Input: part model. Units: mm. Frame: model coordinates. Face numbers are marked on the shaded views. A direction names the side the tool comes from. Coordinates: 2 decimals unless noted, no trailing zeros. Order: outer loops, then holes, each group sorted by start corner. A loop starts at its lowest first (then second) coordinate and runs counter-clockwise, first axis right, second up.
from build123d import *

# Parameters (mm, degrees)
SKETCH_1_W           = 102
SKETCH_1_H           = 54
SKETCH_1_W_2         = 44
SKETCH_1_H_2         = 44
EXTRUDE_1_DEPTH      = 5
SKETCH_2_W           = 102
SKETCH_2_H           = 54
SKETCH_2_W_2         = 98
SKETCH_2_H_2         = 49.988098762
SKETCH_2_W_3         = 44
SKETCH_2_H_3         = 44
SKETCH_2_W_4         = 39.827305616
SKETCH_2_H_4         = 40.011901238
EXTRUDE_2_DEPTH      = 3
SKETCH_3_W           = 106
SKETCH_3_H           = 106
SKETCH_3_W_2         = 102
SKETCH_3_H_2         = 102
EXTRUDE_3_DEPTH      = 30
SKETCH_4_W           = 12
SKETCH_4_H           = 10
SKETCH_4_H_2         = 13
CUT_EXTRUDE_1_DEPTH  = 30
SKETCH_5_W           = 44
SKETCH_5_H           = 44
CUT_EXTRUDE_2_DEPTH  = 3
SKETCH_6_W           = 39.675099194
SKETCH_6_H           = 39.248485224
CUT_EXTRUDE_3_DEPTH  = 87.290021993
SKETCH_8_W           = 39.827305616
SKETCH_8_H           = 40.011901238
SKETCH_8_W_2         = 7.107215528
SKETCH_8_H_2         = 49.988098762
EXTRUDE_5_DEPTH      = 2
EXTRUDE_6_DEPTH      = 2
EXTRUDE_6_DEPTH_BACK = 3
SKETCH_9_W           = 44
SKETCH_9_H           = 44
SKETCH_10_W          = 44
SKETCH_10_H          = 44
CUT_EXTRUDE_5_DEPTH  = 3
SKETCH_11_W          = 39.141831732
SKETCH_11_H          = 39.141831732
CUT_EXTRUDE_6_DEPTH  = 3
SKETCH_12_W          = 10
SKETCH_12_H          = 30
EXTRUDE_7_DEPTH      = 10
SKETCH_13_W          = 3.5
SKETCH_13_H          = 24
CUT_EXTRUDE_7_DEPTH  = 20
CUT_EXTRUDE_8_DEPTH  = 29.999730027
SKETCH_15_W          = 15.5
SKETCH_15_H          = 20.5
CUT_EXTRUDE_9_DEPTH  = 30
SKETCH_18_W          = 102
SKETCH_18_H          = 48
CUT_EXTRUDE_11_DEPTH = 2
CUT_EXTRUDE_12_DEPTH = 124.099226215
EXTRUDE_10_DEPTH     = 6
SKETCH_21_R          = 2
EXTRUDE_11_DEPTH     = 3


with BuildPart() as part:
    # 草图1 → 凸台-拉伸1 (new body)
    with BuildSketch(Plane.XY):
        Polygon((-56.9609375, 55.7890625), (49.0390625, 55.7890625), (49.0390625, -2.2109375), (49.0390625, -50.2109375), (-8.9609375, -50.2109375), (-56.9609375, -50.2109375), (-56.9609375, -2.2109375), align=None)
        with Locations((-3.9609375, 26.7890625)):
            Rectangle(SKETCH_1_W, SKETCH_1_H, mode=Mode.SUBTRACT)
        with Locations((-32.9609375, -26.2109375)):
            Rectangle(SKETCH_1_W_2, SKETCH_1_H_2, mode=Mode.SUBTRACT)
    extrude(amount=EXTRUDE_1_DEPTH)

    # 草图2 → 凸台-拉伸2 (add)
    # profile 1 of 2: a face of its own
    with BuildSketch(Plane(origin=(0, 0, 0), x_dir=(-1, 0, 0), z_dir=(0, 0, -1))):
        with Locations((3.9609375, 26.7890625)):
            Rectangle(SKETCH_2_W, SKETCH_2_H)
        with Locations((3.9609375, 26.795013119)):
            Rectangle(SKETCH_2_W_2, SKETCH_2_H_2, mode=Mode.SUBTRACT)
    # profile 2 of 2: a face of its own
    with BuildSketch(Plane(origin=(0, 0, 0), x_dir=(-1, 0, 0), z_dir=(0, 0, -1))):
        with Locations((32.9609375, -26.2109375)):
            Rectangle(SKETCH_2_W_3, SKETCH_2_H_3)
        with Locations((33.047284692, -26.204986881)):
            Rectangle(SKETCH_2_W_4, SKETCH_2_H_4, mode=Mode.SUBTRACT)
    extrude(amount=-EXTRUDE_2_DEPTH)

    # 草图3 → 凸台-拉伸3 (add)
    with BuildSketch(Plane.XY.offset(5)):
        with Locations((-3.9609375, 2.7890625)):
            Rectangle(SKETCH_3_W, SKETCH_3_H)
        with Locations((-3.9609375, 2.7890625)):
            Rectangle(SKETCH_3_W_2, SKETCH_3_H_2, mode=Mode.SUBTRACT)
    extrude(amount=EXTRUDE_3_DEPTH)

    # 草图4 → 切除-拉伸1 (cut)
    with BuildSketch(Plane(origin=(49.0390625, 0, 0), x_dir=(0, 0, -1), z_dir=(1, 0, 0))):
        with Locations((-9, 44.531190652)):
            Rectangle(SKETCH_4_W, SKETCH_4_H)
        with Locations((-9, 13.608528945)):
            Rectangle(SKETCH_4_W, SKETCH_4_H_2)
    extrude(amount=-CUT_EXTRUDE_1_DEPTH, mode=Mode.SUBTRACT)

    # 草图5 → 切除-拉伸2 (cut)
    with BuildSketch(Plane.XY.offset(5)):
        with Locations((18.871191973, -24.065672965)):
            Rectangle(SKETCH_5_W, SKETCH_5_H)
    extrude(amount=-CUT_EXTRUDE_2_DEPTH, mode=Mode.SUBTRACT)

    # 草图6 → 切除-拉伸3 (cut, through all)
    with BuildSketch(Plane.XY.offset(2)):
        with Locations((19.129543617, -24.247597838)):
            Rectangle(SKETCH_6_W, SKETCH_6_H)
    extrude(amount=-CUT_EXTRUDE_3_DEPTH, mode=Mode.SUBTRACT)

    # 草图8 → 凸台-拉伸5 (add)
    with BuildSketch(Plane(origin=(0, 0, 0), x_dir=(-1, 0, 0), z_dir=(0, 0, -1))):
        with Locations((33.047284692, -26.204986881)):
            Rectangle(SKETCH_8_W, SKETCH_8_H)
        with Locations((3.553607764, 26.795013119)):
            Rectangle(SKETCH_8_W_2, SKETCH_8_H_2)
    extrude(amount=-EXTRUDE_5_DEPTH)

    # 草图9 → 凸台-拉伸6 (add, two sides: drawn at the far end of the back side and taken through both)
    with BuildSketch(Plane.XY.offset(3).offset(-EXTRUDE_6_DEPTH_BACK)):
        with Locations((-32.9609375, -26.2109375)):
            Rectangle(SKETCH_9_W, SKETCH_9_H)
    extrude(amount=EXTRUDE_6_DEPTH + EXTRUDE_6_DEPTH_BACK)

    # 草图10 → 切除-拉伸5 (cut)
    with BuildSketch(Plane.XY.offset(5)):
        with Locations((-27.400759648, -24.065672965)):
            Rectangle(SKETCH_10_W, SKETCH_10_H)
    extrude(amount=-CUT_EXTRUDE_5_DEPTH, mode=Mode.SUBTRACT)

    # 草图11 → 切除-拉伸6 (cut)
    with BuildSketch(Plane.XY.offset(2)):
        with Locations((-27.424705841, -24.087617599)):
            Rectangle(SKETCH_11_W, SKETCH_11_H)
    extrude(amount=-CUT_EXTRUDE_6_DEPTH, mode=Mode.SUBTRACT)

    # 草图12 → 凸台-拉伸7 (add)
    with BuildSketch(Plane(origin=(49.0390625, 0, 0), x_dir=(0, 0, -1), z_dir=(1, 0, 0))):
        with Locations((-25.778359811, 38.789332473)):
            Rectangle(SKETCH_12_W, SKETCH_12_H)
    extrude(amount=-EXTRUDE_7_DEPTH)

    # 草图13 → 切除-拉伸7 (cut)
    with BuildSketch(Plane(origin=(49.0390625, 0, 0), x_dir=(0, 0, -1), z_dir=(1, 0, 0))):
        with Locations((-27.833078142, 37.536383555)):
            Rectangle(SKETCH_13_W, SKETCH_13_H)
    extrude(amount=-CUT_EXTRUDE_7_DEPTH, mode=Mode.SUBTRACT)

    # 草图14 → 切除-拉伸8 (cut)
    with BuildSketch(Plane.XZ.offset(-23.789332473)):
        Polygon((37.906859467, 25.472396685), (38.543242323, 25.472396685), (47.0390625, 20.778359811), (47.0390625, 19.400243598), (37.906859467, 19.400243598), align=None)
    extrude(amount=-CUT_EXTRUDE_8_DEPTH, mode=Mode.SUBTRACT)

    # 草图15 → 切除-拉伸9 (cut)
    with BuildSketch(Plane(origin=(49.0390625, 0, 0), x_dir=(0, 0, -1), z_dir=(1, 0, 0))):
        with Locations((-24.841469183, 4.666763342)):
            Rectangle(SKETCH_15_W, SKETCH_15_H)
    extrude(amount=-CUT_EXTRUDE_9_DEPTH, mode=Mode.SUBTRACT)

    # 草图18 → 切除-拉伸11 (cut)
    with BuildSketch(Plane.XY.offset(5)):
        with Locations((-3.9609375, -24.2109375)):
            Rectangle(SKETCH_18_W, SKETCH_18_H)
    extrude(amount=-CUT_EXTRUDE_11_DEPTH, mode=Mode.SUBTRACT)

    # 草图19 → 切除-拉伸12 (cut, through all)
    with BuildSketch(Plane(origin=(-54.9609375, 0, 0), x_dir=(0, 0, -1), z_dir=(1, 0, 0))):
        with BuildLine():
            Line((-8, -9.636069371), (-6, -9.636069371))
            ThreePointArc((-6, -9.636069371), (-3.878679656, -10.514749028), (-3, -12.636069371))
            Line((-3, -12.636069371), (-3, -36.636069371))
            ThreePointArc((-3, -36.636069371), (-3.878679656, -38.757389715), (-6, -39.636069371))
            Line((-6, -39.636069371), (-8, -39.636069371))
            ThreePointArc((-8, -39.636069371), (-10.121320344, -38.757389715), (-11, -36.636069371))
            Line((-11, -36.636069371), (-11, -12.636069371))
            ThreePointArc((-11, -12.636069371), (-10.121320344, -10.514749028), (-8, -9.636069371))
        make_face()
    extrude(amount=-CUT_EXTRUDE_12_DEPTH, mode=Mode.SUBTRACT)

    # 草图20 → 凸台-拉伸10 (add)
    with BuildSketch(Plane.ZY.offset(56.9609375)):
        with BuildLine():
            Line((3, -36.636069371), (3, -41.845424094))
            Line((3, -41.845424094), (9.180533555, -41.845424094))
            ThreePointArc((9.180533555, -41.845424094), (12.00896068, -40.673851218), (13.180533555, -37.845424094))
            Line((13.180533555, -37.845424094), (13.180533555, -11.076385552))
            ThreePointArc((13.180533555, -11.076385552), (12.00896068, -8.247958428), (9.180533555, -7.076385552))
            Line((9.180533555, -7.076385552), (3, -7.076385552))
            Line((3, -7.076385552), (3, -12.636069371))
            ThreePointArc((3, -12.636069371), (3.878679656, -10.514749028), (6, -9.636069371))
            Line((6, -9.636069371), (8, -9.636069371))
            ThreePointArc((8, -9.636069371), (10.121320344, -10.514749028), (11, -12.636069371))
            Line((11, -12.636069371), (11, -36.636069371))
            ThreePointArc((11, -36.636069371), (10.121320344, -38.757389715), (8, -39.636069371))
            Line((8, -39.636069371), (6, -39.636069371))
            ThreePointArc((6, -39.636069371), (3.878679656, -38.757389715), (3, -36.636069371))
        make_face()
        Polygon((0, -7.076385552), (0, -41.845424094), (3, -41.845424094), (3, -36.636069371), (3, -12.636069371), (3, -7.076385552), align=None)
    extrude(amount=EXTRUDE_10_DEPTH)

    # 草图21 → 凸台-拉伸11 (add)
    # profile 1 of 2: a face of its own
    with BuildSketch(Plane(origin=(0, 0, 0), x_dir=(-1, 0, 0), z_dir=(0, 0, -1))):
        with BuildLine():
            Line((56.9609375, -2.916899347), (64.873289872, -2.916899347))
            ThreePointArc((64.873289872, -2.916899347), (67.701716997, -1.745326471), (68.873289872, 1.083100653))
            Line((68.873289872, 1.083100653), (68.873289872, 4.495024347))
            ThreePointArc((68.873289872, 4.495024347), (67.701716997, 7.323451471), (64.873289872, 8.495024347))
            Line((64.873289872, 8.495024347), (56.9609375, 8.495024347))
            Line((56.9609375, 8.495024347), (56.9609375, -2.916899347))
        make_face()
        with Locations((62.900694294, 2.7890625)):
            Circle(SKETCH_21_R, mode=Mode.SUBTRACT)
    # profile 2 of 2: a face of its own
    with BuildSketch(Plane(origin=(0, 0, 0), x_dir=(-1, 0, 0), z_dir=(0, 0, -1))):
        with BuildLine():
            Line((-60.951414872, 1.083100653), (-60.951414872, 4.495024347))
            ThreePointArc((-60.951414872, 4.495024347), (-59.779841997, 7.323451471), (-56.951414872, 8.495024347))
            Line((-56.951414872, 8.495024347), (-49.0390625, 8.495024347))
            Line((-49.0390625, 8.495024347), (-49.0390625, -2.916899347))
            Line((-49.0390625, -2.916899347), (-56.951414872, -2.916899347))
            ThreePointArc((-56.951414872, -2.916899347), (-59.779841997, -1.745326471), (-60.951414872, 1.083100653))
        make_face()
        with Locations(Location((-54.978819294, 2.7890625, 0), (0, 0, 180))):
            Circle(SKETCH_21_R, mode=Mode.SUBTRACT)
    extrude(amount=-EXTRUDE_11_DEPTH)


solid = part.part
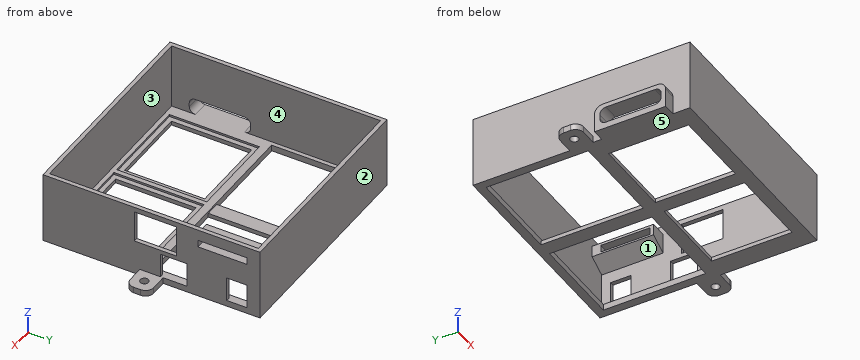
Item 1: Ray query, probe 1 along X at (y, z) = (-19, 29.5); probe 2 along Y at (x, z) = (27.5, 29); probe 3 along X at (y, z) = (32, 26). Return the intervals inside material, ascending.
Response values:
probe 1: x = -56.96 to -54.96, 47.04 to 49.04
probe 2: y = -50.21 to -48.21, 53.79 to 55.79
probe 3: x = -56.96 to -54.96, 39.04 to 49.04
Item 2: Pin query (flat end, axial travel): pin 1 Ø6 at (y, z) = (-24, 26) entering from -X; pin 2 Ø3.5 at (x, z) = (-59.5, 1.5) entering from -Y; pin 3 Ø2 at (y, z) = (-30.5, 8.5) entering from -X. Return the tip coordinate at first contact, or that it passes through.
Response values:
pin 1: stops at x = -56.96
pin 2: stops at y = -41.85
pin 3: stops at x = 47.04
Item 3: Cut plane A-A on x = -13. Return loops of the section in (y, z).
Response values:
outline: (-50.21, 0) - (-43.66, 0) - (-43.66, 2) - (-46.07, 2) - (-46.07, 3) - (-48.21, 3) - (-48.21, 35) - (-50.21, 35) - close; (-4.52, 0) - (1.8, 0) - (1.8, 3) - (-2.07, 3) - (-2.07, 2) - (-4.52, 2) - close; (51.79, 0) - (55.79, 0) - (55.79, 35) - (53.79, 35) - (53.79, 3) - (51.79, 3) - close
Item 4: Draft query along X for the marked faces 4 and 5. Return one class per face: pulls with the +X half, pulls with the -X half, needs draft (parallel to the pull), parting line crosses it, or undercut.
Response values:
face 4: undercut
face 5: needs draft
Item 5: Cut plane C-C on z = 4.5. Return loops of the section in (x, y).
Response values:
outline: (-62.96, -41.85) - (-56.96, -41.85) - (-56.96, -50.21) - (49.04, -50.21) - (49.04, 7.11) - (47.04, 7.11) - (47.04, -48.21) - (-54.96, -48.21) - (-54.96, -39.23) - (-62.96, -39.23) - close; (-62.96, -10.04) - (-54.96, -10.04) - (-54.96, 53.79) - (47.04, 53.79) - (47.04, 49.53) - (49.04, 49.53) - (49.04, 55.79) - (-56.96, 55.79) - (-56.96, -7.08) - (-62.96, -7.08) - close; (47.04, 20.11) - (49.04, 20.11) - (49.04, 39.53) - (47.04, 39.53) - close
Item 6: Cut plane D-D on y = -26.5. Return loops of the section in (x, z).
Response values:
outline: (-62.96, 0) - (-47, 0) - (-47, 2) - (-49.4, 2) - (-49.4, 3) - (-62.96, 3) - close; (-62.96, 11) - (-54.96, 11) - (-54.96, 35) - (-56.96, 35) - (-56.96, 13.18) - (-62.96, 13.18) - close; (-7.85, 0) - (-0.71, 0) - (-0.71, 2) - (-3.13, 2) - (-3.13, 3) - (-5.4, 3) - (-5.4, 2) - (-7.85, 2) - close; (38.97, 0) - (49.04, 0) - (49.04, 35) - (47.04, 35) - (47.04, 3) - (40.87, 3) - (40.87, 2) - (38.97, 2) - close
Item 7: Cut plane B-B on y = 10. Return loops of the section in (x, z), then the cut area to 3 significant figures.
Response values:
outline: (-56.96, 0) - (-52.96, 0) - (-52.96, 3) - (-54.96, 3) - (-54.96, 35) - (-56.96, 35) - close; (-7.11, 0) - (0, 0) - (0, 2) - (-7.11, 2) - close; (45.04, 0) - (49.04, 0) - (49.04, 3) - (45.04, 3) - close; (47.04, 15) - (49.04, 15) - (49.04, 17.09) - (47.04, 17.09) - close; (47.04, 32.59) - (49.04, 32.59) - (49.04, 35) - (47.04, 35) - close
area: 111 mm2
Item 8: Access query for the marked faces 1, 2 and 3. Directions: +Z, -Z, +X, -X, +Y, -Y. A direction counts if a zero-diameter tool reaches every point of the face in a straight line with its end or side. Return the directions, or none.
Response values:
face 1: none
face 2: +Z, -Z, +X, -X, +Y
face 3: +Z
